Work out the finished part from the listing and answer in its coordinate system (mm). A direction names the side the tool comes from. Give positions to 0.01 mm unless a question says otherwise; leave off trailing zeros. Loops run counter-clockwise (first coordinate to the right, second up) from the corner with the lowest first, then second, coordinate; pieces in that order, holes last. Notation, with made-up numbers: M 61.25,17 L 71.25,17 A26 ccw 71.25,36 Z; hole C -18,26 d6. An arc over 180 degrees is marked long. Answer in a Markdown table with one row per item. Add a question column.
from build123d import *

# Parameters (mm, degrees)
BOSS_EXTRUDE1_DEPTH     = 3.175
CUT_EXTRUDE1_DEPTH      = 78.429520372
MIRROR2_COPY_1_DEPTH    = 78.429520372
SKETCH4_W               = 138
SKETCH4_H               = 20
BOSS_EXTRUDE3_DEPTH     = 3.175
CUT_EXTRUDE2_DEPTH      = 87.459994362
CUT_EXTRUDE2_DEPTH_BACK = 87.459994362
SKETCH5_W               = 80
SKETCH5_H               = 5
FILLET1_R               = 2.5
SKETCH6_W               = 3.5
SKETCH6_H               = 1
CUT_EXTRUDE3_DEPTH      = 87.459994362
SKETCH10_W              = 40
SKETCH10_H              = 20
CUT_EXTRUDE4_DEPTH      = 87.459994362
SKETCH11_R              = 1
SKETCH11_W              = 20
SKETCH11_H              = 3.18
CUT_EXTRUDE5_DEPTH      = 87.459994362
SKETCH12_R              = 1.25
CUT_EXTRUDE6_DEPTH      = 87.459994362
MIRROR5_COPY_1_SKETCH_R = 1
MIRROR5_COPY_1_SKETCH_W = 20
MIRROR5_COPY_1_SKETCH_H = 3.18
MIRROR5_COPY_1_DEPTH    = 87.459994362
MIRROR5_COPY_2_SKETCH_R = 1.25
MIRROR5_COPY_2_DEPTH    = 87.459994362
SKETCH13_R              = 3.75
SKETCH13_R_2            = 7.9375
CUT_EXTRUDE7_DEPTH      = 87.459994362
SKETCH14_R              = 1.45
CUT_EXTRUDE8_DEPTH      = 87.459994362


with BuildPart() as part:
    # Sketch1 → Boss-Extrude1 (new body)
    with BuildSketch(Plane.XY):
        Polygon((-69, -10), (-69, -27), (69, -27), (69, -10), (72.5, -10), (72.5, 10), (69, 10), (69, 25), (-69, 25), (-69, 10), (-72.5, 10), (-72.5, -10), align=None)
    extrude(amount=-BOSS_EXTRUDE1_DEPTH)

    # Sketch2 → Cut-Extrude1 (cut, symmetric)
    with BuildSketch(Plane.XY):
        Polygon((-69, 19.5), (-65, 19.5), (-65, 20.5), (-61.5, 20.5), (-61.5, 16.5), (-65, 16.5), (-65, 17.5), (-69, 17.5), align=None)
    cut_extrude1 = extrude(amount=CUT_EXTRUDE1_DEPTH, both=True, mode=Mode.SUBTRACT)

    # Mirror1: Cut-Extrude1 across plane
    add(cut_extrude1.mirror(Plane.ZY), mode=Mode.SUBTRACT)

    # Mirror2: Cut-Extrude1 across plane
    add(cut_extrude1.mirror(Plane.ZX), mode=Mode.SUBTRACT)

    # Mirror2 copy 1 sketch → Mirror2 copy 1 (cut, symmetric)
    with BuildSketch(Plane(origin=(0, 0, 0), x_dir=(-1, 0, 0), z_dir=(0, 0, 1))):
        Polygon((-69, 19.5), (-65, 19.5), (-65, 20.5), (-61.5, 20.5), (-61.5, 16.5), (-65, 16.5), (-65, 17.5), (-69, 17.5), align=None)
    extrude(amount=MIRROR2_COPY_1_DEPTH, both=True, mode=Mode.SUBTRACT)

    # Sketch4 → Boss-Extrude3 (add)
    with BuildSketch(Plane.XY):
        with Locations((0, -37)):
            Rectangle(SKETCH4_W, SKETCH4_H)
    extrude(amount=-BOSS_EXTRUDE3_DEPTH)

    # Sketch5 → Cut-Extrude2 (cut, two sides: drawn at the far end of the back side and taken through both)
    with BuildSketch(Plane.XY.offset(-CUT_EXTRUDE2_DEPTH_BACK)):
        with Locations((0, 22.5)):
            Rectangle(SKETCH5_W, SKETCH5_H)
    extrude(amount=CUT_EXTRUDE2_DEPTH + CUT_EXTRUDE2_DEPTH_BACK, mode=Mode.SUBTRACT)

    # Fillet1
    fillet1_edges = [part.edges().sort_by_distance(p)[0] for p in [
        (40, 20, -1.5875),
        (-40, 20, -1.5875),
    ]]
    fillet(fillet1_edges, radius=FILLET1_R)
    fillet1_2_edges = [part.edges().sort_by_distance(p)[0] for p in [
        (40, 25, -1.5875),
        (-40, 25, -1.5875),
    ]]
    fillet(fillet1_2_edges, radius=FILLET1_R - 0.0001)  # a hair under: the kernel refuses the full size

    # Sketch6 → Cut-Extrude3 (cut, symmetric)
    with BuildSketch(Plane.XY):
        with Locations((63.25, -46.5)):
            Rectangle(SKETCH6_W, SKETCH6_H)
    cut_extrude3 = extrude(amount=CUT_EXTRUDE3_DEPTH, both=True, mode=Mode.SUBTRACT)

    # Mirror3: Cut-Extrude3 across plane
    add(cut_extrude3.mirror(Plane.ZY), mode=Mode.SUBTRACT)

    # Sketch10 → Cut-Extrude4 (cut, through all)
    with BuildSketch(Plane(origin=(0, 0, -3.175), x_dir=(-1, 0, 0), z_dir=(0, 0, -1))):
        with Locations((33.5, -5)):
            Rectangle(SKETCH10_W, SKETCH10_H)
    cut_extrude4 = extrude(amount=-CUT_EXTRUDE4_DEPTH, mode=Mode.SUBTRACT)

    # Sketch11 → Cut-Extrude5 (cut, through all)
    with BuildSketch(Plane(origin=(0, 0, -3.175), x_dir=(-1, 0, 0), z_dir=(0, 0, -1))):
        with Locations((15, -20.41)):
            Circle(SKETCH11_R)
        with Locations((52, -20.41)):
            Circle(SKETCH11_R)
        with Locations((33.5, -20.41)):
            Rectangle(SKETCH11_W, SKETCH11_H)
    cut_extrude5 = extrude(amount=-CUT_EXTRUDE5_DEPTH, mode=Mode.SUBTRACT)

    # Sketch12 → Cut-Extrude6 (cut, through all)
    with BuildSketch(Plane(origin=(0, 0, -3.175), x_dir=(-1, 0, 0), z_dir=(0, 0, -1))):
        with Locations((8.75, -10)):
            Circle(SKETCH12_R)
        with Locations((58.25, -10)):
            Circle(SKETCH12_R)
    cut_extrude6 = extrude(amount=-CUT_EXTRUDE6_DEPTH, mode=Mode.SUBTRACT)

    # Mirror4: Cut-Extrude5, Cut-Extrude6 across plane
    add(cut_extrude5.mirror(Plane.ZX.offset(-5)), mode=Mode.SUBTRACT)
    add(cut_extrude6.mirror(Plane.ZX.offset(-5)), mode=Mode.SUBTRACT)

    # Mirror5: Cut-Extrude4, Cut-Extrude5, Cut-Extrude6 across plane
    add(cut_extrude4.mirror(Plane.ZY), mode=Mode.SUBTRACT)
    add(cut_extrude5.mirror(Plane.ZY), mode=Mode.SUBTRACT)
    add(cut_extrude6.mirror(Plane.ZY), mode=Mode.SUBTRACT)

    # Mirror5 copy 1 sketch → Mirror5 copy 1 (cut, through all)
    with BuildSketch(Plane(origin=(0, -10, -3.175), x_dir=(1, 0, 0), z_dir=(0, 0, -1))):
        with Locations((15, -20.41)):
            Circle(MIRROR5_COPY_1_SKETCH_R)
        with Locations((52, -20.41)):
            Circle(MIRROR5_COPY_1_SKETCH_R)
        with Locations((33.5, -20.41)):
            Rectangle(MIRROR5_COPY_1_SKETCH_W, MIRROR5_COPY_1_SKETCH_H)
    extrude(amount=-MIRROR5_COPY_1_DEPTH, mode=Mode.SUBTRACT)

    # Mirror5 copy 2 sketch → Mirror5 copy 2 (cut, through all)
    with BuildSketch(Plane(origin=(0, -10, -3.175), x_dir=(1, 0, 0), z_dir=(0, 0, -1))):
        with Locations((8.75, -10)):
            Circle(MIRROR5_COPY_2_SKETCH_R)
        with Locations((58.25, -10)):
            Circle(MIRROR5_COPY_2_SKETCH_R)
    extrude(amount=-MIRROR5_COPY_2_DEPTH, mode=Mode.SUBTRACT)

    # Sketch13 → Cut-Extrude7 (cut, through all)
    with BuildSketch(Plane.XY):
        with Locations((-15.875, -35)):
            Circle(SKETCH13_R)
        with Locations((15.875, -35)):
            Circle(SKETCH13_R_2)
    extrude(amount=-CUT_EXTRUDE7_DEPTH, mode=Mode.SUBTRACT)

    # Sketch14 → Cut-Extrude8 (cut, through all)
    with BuildSketch(Plane.XY):
        with Locations((-23.375, -35)):
            Circle(SKETCH14_R)
        with Locations((-15.875, -27.5)):
            Circle(SKETCH14_R)
        with Locations((-8.375, -35)):
            Circle(SKETCH14_R)
        with Locations((-15.875, -42.5)):
            Circle(SKETCH14_R)
    extrude(amount=-CUT_EXTRUDE8_DEPTH, mode=Mode.SUBTRACT)


solid = part.part
(1) Which of the six approach directions +Z, -Z, +X, -X, +Y, -Y give full straight-line access (tool end or side, diameter ignored) to faces 5 (the face through (-1, -10, 0)), 6 (the face through (23.5, -20, -2)), 7 (the face through (63, -46, -2))?
(2) Section A-A, the plane z = -0.5 is taken. State how many separate pieces and enclosed holes the cut face has, and give its area (3 significant figures).
(3) Section B-B, the plane y = 14 is taken. Determine the outline of the cut face in (x, z) (3 decimals).
(4) Consider line 1 along X through (y, z) = (-7.5, -1.3); line 2 along Y through (x, z) = (-58.25, -2.05); line 3 along X through (y, z) = (22.5, -0.7). Determine where each line is inside the solid, lowest interval first. Write a range as from..to.
(5) Each of these flat-tipped pins is pushed along its axis until it touches: P1, Ø2.5, axis at x = 52, y = -20.41, coming from the +Z side; P2, Ø0.5, axis at y = 17, z = -2.5, coming from the +X side; P3, Ø1, axis at y = 18.5, z = -1.5, coming from the -X side; P4, Ø1.6, axis at x = -33.5, z = -1.5, coming from the +Y side. Where does it stop, or does it pass through?
(6) The mould has two halves that part along X. Classify faces 1 (the face through (-63, 16.5, -2)), 2 (the face through (67, -47, -2)), 3 (the face through (69, -33, -2)), 4 (the face through (39.248, 20.713, -1.565)): pulls with the +X half, pulls with the -X half, needs draft (parallel to the pull), parting line crosses it, or undercut.
Numbers:
| question | item | result |
|---|---|---|
| 1 | face 5 | +Z, +X, -X, +Y, -Y |
| 1 | face 6 | +Z, -Z |
| 1 | face 7 | +Z, -Z, -Y |
| 2 | separate pieces | 1 |
| 2 | enclosed holes | 28 |
| 2 | area | 7,390 mm² |
| 3 | outline | M -69,-3.175 L 69,-3.175 L 69,0 L -69,0 Z |
| 4 | line 1 | x = -72.5..-53.5, -13.5..13.5, 53.5..72.5 |
| 4 | line 2 | y = -47..-11.25, -8.75..-1.25, 1.25..25 |
| 4 | line 3 | x = -69..-40, 40..69 |
| 5 | P1 | stops at z = 0 |
| 5 | P2 | stops at x = 69 |
| 5 | P3 | stops at x = -61.5 |
| 5 | P4 | stops at y = 20 |
| 6 | face 1 | undercut |
| 6 | face 2 | needs draft |
| 6 | face 3 | pulls with the +X half |
| 6 | face 4 | undercut |
